Design review of the part built by this model. Coordinates are the model's own, in mm. A direction names the side the tool comes from. Coordinates: 2 decimals unless noted, no trailing zeros. Loops run counter-clockwise (first coordinate to the right, second up) from the corner with the lowest first, then second, coordinate; pieces in that order, holes last. Notation, with made-up numbers: (19, 24.25) -> (76, 24.25) arc R14 ccw to (76, 31.25) -> close; hole circle Ø3 at (21, 88.25). An arc over 180 degrees is marked (long way). One line per item, written item: value. Start each with the question number.
1. For probe 1 along Z at (x, y) = (-51, -26) (3 decimals); probe 2 along X at (y, z) = (2, 114.5), list the stretches that pass through material, from the lowest coordinate up.
2. Add section A-A on x = 15. Write out the cut boundary in (y, z) (3 decimals), plus the area to 3 significant figures.
3. Insertion check: pin 1 (4 mm diameter, centred on x = 41, z = 121, fed in from -Y); pin 2 (5 mm diameter, centred on y = -20, z = 3, fed in from +X); pin 3 (5 mm diameter, centred on x = -2.5, y = 14.5, fed in from +Z). Each pin has a flat end and moves straight along its axis. Give the tip position at first contact, or say it passes through.
4. Add section B-B on y = -21. Write out the cut boundary in (x, z).
5. Draft analysis for pull direction X (two halves, no side actions). For faces 1 (the flat face through (38, -25, 94)), 2 (the flat face through (63, -27, 43)), 3 (the cylindrical face through (-48.099, -27.465, 48.173)), state which applies: pulls with the +X half, pulls with the -X half, needs draft (parallel to the pull), parting line crosses it, or undercut.
6. Machinability: for faces 4 (the flat face through (0, 25, 89)), 5 (the flat face through (-57.1, -25, 145.9)), 6 (the flat face through (57, -25, 46)), 7 (the flat face through (5, -18, 3)), which of the approach directions +Z, -Z, +X, -X, +Y, -Y give a long, thin tool a straight path to every point of the face, cutting with its end or side? Answer none if there is none.
7. Add section C-C on z = 52. Write out the cut boundary in (x, y).
8. Add section D-D on x = 51.18. Write out the cut boundary in (y, z) (3 decimals).
```python
from build123d import *

# Parameters (mm, degrees)
F1_DEPTH  = 6.35
F2_W      = 50
F2_H      = 180
F3_DEPTH  = 6.35
F4_W      = 50
F4_H      = 180
F5_DEPTH  = 6.35
F6_W      = 70
F6_H      = 163.65
F7_DEPTH  = 6.35
F8_R      = 5.75
F8_W      = 6.35
F8_H      = 12.7
F8_W_2    = 30
F9_DEPTH  = 5
F11_DEPTH = 5


# Not quite as in the source:
# - a feature names something its author has since deleted; it is built from what else it names


with BuildPart() as f1:
    # F0 (on Top) → F1 (new body)
    with BuildSketch(Plane.XY):
        with BuildLine():
            Line((35, -25), (35, 25))
            Line((35, 25), (-35, 25))
            Line((-35, 25), (-35, -25))
            Line((-35, -25), (-5, -25))
            Line((-5, -25), (-5, -11.8))
            ThreePointArc((-5, -11.8), (0, -6.8), (5, -11.8))
            Line((5, -11.8), (5, -25))
            Line((5, -25), (35, -25))
        make_face()
    extrude(amount=F1_DEPTH)

    # F2 (on face) → F3 (join)
    with BuildSketch(Plane(origin=(-35, 0, 0), x_dir=(0, -1, 0), z_dir=(-1, 0, 0))):
        with Locations((0, 90)):
            Rectangle(F2_W, F2_H)
    extrude(amount=F3_DEPTH)

    # F4 (on face) → F5 (join)
    with BuildSketch(Plane.YZ.offset(35)):
        with Locations((0, 90)):
            Rectangle(F4_W, F4_H)
    extrude(amount=F5_DEPTH)

    # F6 (on face) → F7 (join)
    with BuildSketch(Plane(origin=(0, 25, 0), x_dir=(-1, 0, 0), z_dir=(0, 1, 0))):
        with Locations((0, 88.175)):
            Rectangle(F6_W, F6_H)
        Polygon((-41.35, 0), (41.35, 0), (41.35, 170), (35, 170), (35, 6.35), (-35, 6.35), (-35, 170), (-41.35, 170), align=None)
    extrude(amount=F7_DEPTH)

    # F8 (on face) → F9 (join)
    with BuildSketch(Plane.XZ.offset(25)):
        Polygon((-63, 30.625), (-5, 30.625), (-5, 43.325), (-5, 56.025), (-63, 56.025), align=None)
        with Locations((-51.19, 43.325)):
            Circle(F8_R, mode=Mode.SUBTRACT)
        Polygon((-5, 30.625), (5, 30.625), (5, 43.325), (5, 56.025), (-5, 56.025), (-5, 43.325), align=None)
        Polygon((41.35, 43.325), (41.35, 30.625), (63, 30.625), (63, 56.025), (41.35, 56.025), align=None)
        with BuildLine():
            ThreePointArc((56.94, 43.325), (51.19, 37.575), (45.44, 43.325))
            ThreePointArc((45.44, 43.325), (51.19, 49.075), (56.94, 43.325))
        make_face(mode=Mode.SUBTRACT)
        with Locations((38.175, 49.675)):
            Rectangle(F8_W, F8_H)
        with Locations((38.175, 36.975)):
            Rectangle(F8_W, F8_H)
        with Locations((20, 36.975)):
            Rectangle(F8_W_2, F8_H)
        with Locations((20, 49.675)):
            Rectangle(F8_W_2, F8_H)
    extrude(amount=F9_DEPTH)

    # F10 (on face) → F11 (join)
    with BuildSketch(Plane.XZ.offset(30)):
        Polygon((-63, 132.995), (-51.19, 132.995), (63, 132.995), (63, 158.395), (-63, 158.395), align=None)
        with BuildLine():
            ThreePointArc((-45.44, 145.695), (-47.1241360082, 141.6291360082), (-51.19, 139.945))
            ThreePointArc((-51.19, 139.945), (-55.2558639918, 149.7608639918), (-45.44, 145.695))
        make_face(mode=Mode.SUBTRACT)
        with BuildLine():
            ThreePointArc((56.93, 145.695), (51.18, 139.945), (45.43, 145.695))
            ThreePointArc((45.43, 145.695), (51.18, 151.445), (56.93, 145.695))
        make_face(mode=Mode.SUBTRACT)
    extrude(amount=-F11_DEPTH)


solid = f1.part
```
Worked answers:
1. probe 1: z = 30.625 to 37.578, 49.072 to 56.025, 132.995 to 139.948, 151.442 to 158.395
1. probe 2: x = -41.35 to -35, 35 to 41.35
2. outline: (-30, 30.625) -> (-25, 30.625) -> (-25, 56.025) -> (-30, 56.025) -> close; (-30, 132.995) -> (-25, 132.995) -> (-25, 158.395) -> (-30, 158.395) -> close; (-25, 0) -> (31.35, 0) -> (31.35, 170) -> (25, 170) -> (25, 6.35) -> (-25, 6.35) -> close
2. area: 1,650 mm²
3. pin 1: stops at y = -25
3. pin 2: stops at x = 41.35
3. pin 3: stops at z = 6.35
4. outline: (-41.35, 0) -> (-5, 0) -> (-5, 6.35) -> (-35, 6.35) -> (-35, 180) -> (-41.35, 180) -> close; (5, 0) -> (41.35, 0) -> (41.35, 180) -> (35, 180) -> (35, 6.35) -> (5, 6.35) -> close
5. face 1: needs draft
5. face 2: pulls with the +X half
5. face 3: undercut
6. face 4: +Z
6. face 5: +Z, -Z, -X, +Y
6. face 6: +Z, -Z, +X, +Y
6. face 7: +Z, -Z, -Y
7. outline: (-63, -30) -> (63, -30) -> (63, -25) -> (41.35, -25) -> (41.35, 31.35) -> (-41.35, 31.35) -> (-41.35, -25) -> (-63, -25) -> close; hole (-35, -25) -> (35, -25) -> (35, 25) -> (-35, 25) -> close
8. outline: (-30, 30.625) -> (-25, 30.625) -> (-25, 37.575) -> (-30, 37.575) -> close; (-30, 49.075) -> (-25, 49.075) -> (-25, 56.025) -> (-30, 56.025) -> close; (-30, 132.995) -> (-25, 132.995) -> (-25, 139.945) -> (-30, 139.945) -> close; (-30, 151.445) -> (-25, 151.445) -> (-25, 158.395) -> (-30, 158.395) -> close
